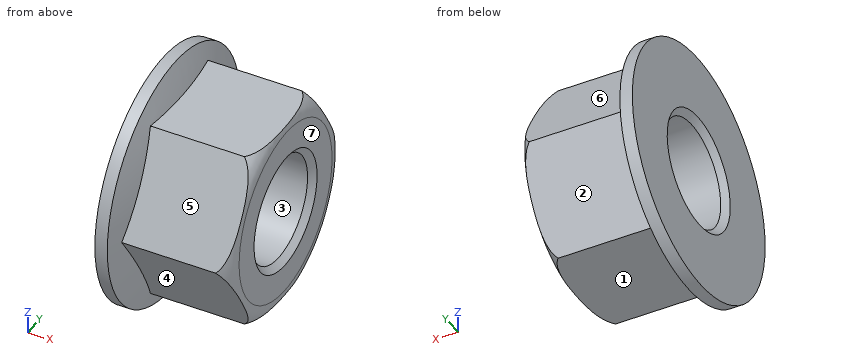
```python
from build123d import *

# Parameters (mm, degrees)
EXTRUSION1_DEPTH        = 10
ESQUISSE4_R             = 4.25
ENL_V_MAT_EXTRU_2_DEPTH = 10
CHANFREIN1_SIZE         = 0.5


with BuildPart() as part:
    # Esquisse1 → Extrusion1 (new body)
    with BuildSketch(Plane(origin=(0, 0, 0), x_dir=(0, 0, -1), z_dir=(1, 0, 0))):
        Polygon((0, 8.660254038), (-7.5, 4.330127019), (-7.5, -4.330127019), (0, -8.660254038), (7.5, -4.330127019), (7.5, 4.330127019), align=None)
    extrude(amount=EXTRUSION1_DEPTH)

    # Esquisse2 → Enlèvement de matière-Révolution1 (revolve, cut)
    with BuildSketch(Plane.XY, mode=Mode.PRIVATE) as enl_vement_de_mati_re_r_volution1_sk:
        with BuildLine():
            Line((10, 8.660254038), (9, 8.660254038))
            ThreePointArc((9, 8.660254038), (9.730692812, 7.969077328), (10, 7))
            Line((10, 7), (10, 8.660254038))
        make_face()
    revolve(enl_vement_de_mati_re_r_volution1_sk.sketch.rotate(Axis((0, 0, 0), (1, 0, 0)), 90), axis=Axis((0, 0, 0), (1, 0, 0)), mode=Mode.SUBTRACT)  # turned: the seam where the file's is

    # Esquisse3 → Révolution1 (revolve)
    with BuildSketch(Plane.XY, mode=Mode.PRIVATE) as r_volution1_sk:
        with BuildLine():
            Line((0, 0), (0, 10))
            Line((0, 10), (1, 10))
            ThreePointArc((1, 10), (2.283685542, 5.073059362), (2.715728753, 0))
            Line((2.715728753, 0), (0, 0))
        make_face()
    revolve(r_volution1_sk.sketch.rotate(Axis((0, 0, 0), (1, 0, 0)), 180), axis=Axis((0, 0, 0), (1, 0, 0)))  # turned: the seam where the file's is

    # Esquisse4 → Enlèv. mat.-Extru.2 (cut)
    with BuildSketch(Plane(origin=(0, 0, 0), x_dir=(0, 0, -1), z_dir=(1, 0, 0))):
        Circle(ESQUISSE4_R)
    extrude(amount=ENL_V_MAT_EXTRU_2_DEPTH, mode=Mode.SUBTRACT)

    # Chanfrein1
    chanfrein1_edges = [part.edges().sort_by_distance(p)[0] for p in [
        (0, 0, 4.25),
        (10, 0, 4.25),
    ]]
    chamfer(chanfrein1_edges, length=CHANFREIN1_SIZE)


solid = part.part
```
The model under review builds one solid part; all positions refer to its coordinate system, in mm. Face numbers are marked on the shaded views. A direction names the side the tool comes from. Round coordinates to 2 decimals unless told otherwise and drop trailing zeros. Order: outer loops, then holes, each group sorted by start corner. A loop starts at its lowest first (then second) coordinate and runs counter-clockwise, first axis right, second up.
(1) Take a section at A-A, the plane y = 0. State the section outline as (x, z) points.
Working result:
outline: (0, -10) - (1, -10) arc R30 ccw to (1.76, -7.5) - (9.93, -7.5) arc R1.88 ccw to (10, -7) - (10, -4.75) - (9.5, -4.25) - (0.5, -4.25) - (0, -4.75) - close; (0, 4.75) - (0.5, 4.25) - (9.5, 4.25) - (10, 4.75) - (10, 7) arc R1.88 ccw to (9.93, 7.5) - (1.76, 7.5) arc R30 ccw to (1, 10) - (0, 10) - close
(2) Mouldability with a two-part tool opening along Y and no side actions: class the marked faces 1, 2, 3 and 4 as released by +Y, released by -Y, zero draft, split by the parting line, or undercut.
Working result:
face 1: zero draft
face 2: released by +Y
face 3: undercut
face 4: released by -Y
(3) Tool access review of the marked faces 5, 6 and 7: name each direction out of +Z, -Z, +X, -X, +Y, -Y from which nothing blocks a thin tool from reaching the whole face with its end or side.
Working result:
face 5: +Z, +X, -Y
face 6: +Z, +X, +Y
face 7: +Z, -Z, +X, +Y, -Y
(4) For P1, Ø4, axis at x = 7.5, z = 7, coming from the +Y side; P2, Ø3, axis at x = 8.5, y = 7, coming from the +Z side; P3, Ø1, axis at y = 0.5, z = 7.5, coming from the -X side; P4, Ø5, axis at x = 7.5, z = -6.5, coming from the -Y side, all flat-tipped, find the tip position at first contact; note any pin that passes through.
Working result:
P1: stops at y = 5.77
P2: stops at z = 5.47
P3: stops at x = 0
P4: stops at y = -6.35
(5) Take a section at B-B, the plane x = 6.75. State the section outline as (y, z) points, plus the area to 3 significant figures.
Working result:
outline: (-8.66, 0) - (-4.33, -7.5) - (4.33, -7.5) - (8.66, 0) - (4.33, 7.5) - (-4.33, 7.5) - close; hole circle Ø8.5 at (0, 0)
area: 138 mm2
(6) Wall thickness on L1, parallel to Z at x = 2.5, y = -0.25; L2, parallel to Y at x = 9.75, z = -3; L3, parallel to Y at x = 3.25, z = -3.5: over which ranges is each line inside the solid? List them lowest first.
Working result:
L1: z = -7.5 to -4.24, 4.24 to 7.5
L2: y = -6.93 to -3.35, 3.35 to 6.93
L3: y = -6.64 to -2.41, 2.41 to 6.64
